Can you work these out from the model? Positions are in its coordinate system, mm. Face numbers are marked on the shaded views. A direction names the side the tool comes from. Coordinates: 2 decimals unless noted, no trailing zeros. Loops run counter-clockwise (first coordinate to the right, second up) from the corner with the lowest first, then second, coordinate; pieces in that order, holes last. Notation, with made-up numbers: (5, 31) -> (64, 31) arc R10 ccw to (64, 35) -> close; hole circle Ø7 at (-34.5, 77). An arc over 180 degrees is marked (long way). Use one line per item in the form item = value. Start each with the question number.
(1) On a 3-axis mill with a long thin cutter (end or side, diameter ignored), from which of +Z, -Z, +X, -X, +Y, -Y can I reach the whole of each face in a straight line? I mean the marked faces 4, 5, 6 and 7. Say none if no direction works.
(2) Imagine slicing it at A-A (y = -16). List the corners of the cut face in (x, z) for me, plus the area to 3 significant figures.
(3) I'm going to push flat-ended pins straight in: pin 1 (3 mm diameter, centred on y = -11, z = 16.01, fed in from -X); pin 2 (4 mm diameter, centred on y = -12.5, z = 12, fed in from +X); pin 3 (2 mm diameter, centred on x = 23, y = -13.5, fed in from +Z). Where does each tip first touch, or does it pass through?
(4) Thinking about a two-plate mould opening in X: for the marked faces 1, 2 and 3, which applies, released by +X, released by -X, zero draft, split by the parting line, or undercut?
(5) Imagine slicing it at C-C (x = 28). List the corners of the cut face in (y, z) for me.
(6) Imagine slicing it at B-B (z = 8). List the corners of the cut face in (x, y) for me, plus the area to 3 significant figures.
(7) Imagine slicing it at D-D (y = -11). List the corners of the cut face in (x, z) for me, plus the area to 3 significant figures.
(8) I need wall thicknesses on line 1 (X direction, y = -9.5, z = 23.5); line 2 (Z direction, x = 29.5, y = -10.75); line 3 (X direction, y = -2.5, z = 4.5). Which ranges of each line are inside material? Lowest first, please. Write a range as [from, to].
```python
from build123d import *

# Parameters (mm, degrees)
F0_W      = 50
F0_H      = 32
F1_DEPTH  = 24
F2_SIZE   = 4.5
F3_W      = 64.6181842312
F3_H      = 72.6516954601
F4_DEPTH  = 6.5
F6_DEPTH  = 13
F7_R      = 1.4
F8_DEPTH  = 5
F9_R      = 1.4
F10_DEPTH = 5
F11_R     = 1.4
F12_DEPTH = 5
F13_R     = 1.4
F14_DEPTH = 5
F15_R     = 1
F16_DEPTH = 5
F17_R     = 1
F18_DEPTH = 5
F19_R     = 1
F20_DEPTH = 5
F21_R     = 1
F22_DEPTH = 5
F23_R     = 1.1
F24_DEPTH = 25.4
F25_R     = 1.25
F26_DEPTH = 25.4
F27_R     = 1.25
F28_DEPTH = 25.4
F30_DEPTH = 25.4
F32_DEPTH = 25.4


# Not quite as in the source:
# - a feature names something its author has since deleted; it is built from what else it names


with BuildPart() as f1:
    # F0 (on Front) → F1 (new body)
    with BuildSketch(Plane.XZ):
        with Locations((25, 16)):
            Rectangle(F0_W, F0_H)
    extrude(amount=F1_DEPTH)

    # F2
    f2_edges = [f1.edges().sort_by_distance(p)[0] for p in [
        (50, -12, 0),
        (50, -12, 32),
        (50, 0, 16),
        (50, -24, 16),
        (0, -12, 32),
        (25, 0, 32),
        (25, -24, 32),
        (0, -12, 0),
        (0, 0, 16),
        (0, -24, 16),
        (25, 0, 0),
        (25, -24, 0),
    ]]
    chamfer(f2_edges, length=F2_SIZE)

    # F3 (on face) → F4 (cut)
    with BuildSketch(Plane.XZ.offset(24)):
        with Locations((22.701323498, 16.0673912615)):
            Rectangle(F3_W, F3_H)
    extrude(amount=-F4_DEPTH, mode=Mode.SUBTRACT)

    # F5 (on face) → F6 (cut)
    with BuildSketch(Plane.XZ.offset(17.5)):
        Polygon((4.5, 30), (2, 27.5), (2, 4.5), (4.5, 2), (45.5, 2), (48, 4.5), (48, 27.5), (45.5, 30), align=None)
    extrude(amount=-F6_DEPTH, mode=Mode.SUBTRACT)

    # F7 (on face) → F8 (join)
    with BuildSketch(Plane(origin=(38.75, 0, 38.75), x_dir=(0, 1, 0), z_dir=(0.7071067812, 0, 0.7071067812))):
        with Locations((-13.25, -12.7279220614)):
            Circle(F7_R)
        with Locations((-8.75, -12.7279220614)):
            Circle(F7_R)
    extrude(amount=F8_DEPTH)

    # F9 (on face) → F10 (join)
    with BuildSketch(Plane(origin=(22.75, 0, -22.75), x_dir=(0, 1, 0), z_dir=(0.7071067812, 0, -0.7071067812))):
        with Locations((-13.25, 35.3553390593)):
            Circle(F9_R)
        with Locations((-8.75, 35.3553390593)):
            Circle(F9_R)
    extrude(amount=F10_DEPTH)

    # F11 (on face) → F12 (join)
    with BuildSketch(Plane(origin=(2.25, 0, 2.25), x_dir=(0, -1, 0), z_dir=(-0.7071067812, 0, -0.7071067812))):
        with Locations((13.25, 0)):
            Circle(F11_R)
        with Locations((8.75, 0)):
            Circle(F11_R)
    extrude(amount=F12_DEPTH)

    # F13 (on face) → F14 (join)
    with BuildSketch(Plane(origin=(-13.75, 0, 13.75), x_dir=(0, -1, 0), z_dir=(-0.7071067812, 0, 0.7071067812))):
        with Locations((8.75, 22.6343975133)):
            Circle(F13_R)
        with Locations((13.25, 22.6343975133)):
            Circle(F13_R)
    extrude(amount=F14_DEPTH)

    # F15 (on face) → F16 (cut)
    with BuildSketch(Plane(origin=(42.2855339059, 0, 42.2855339059), x_dir=(0, 1, 0), z_dir=(0.7071067812, 0, 0.7071067812))):
        with Locations((-13.25, -12.7279220614)):
            Circle(F15_R)
        with Locations((-8.75, -12.7279220614)):
            Circle(F15_R)
    extrude(amount=-F16_DEPTH, mode=Mode.SUBTRACT)

    # F17 (on face) → F18 (cut)
    with BuildSketch(Plane(origin=(26.2855339059, 0, -26.2855339059), x_dir=(0, 1, 0), z_dir=(0.7071067812, 0, -0.7071067812))):
        with Locations((-13.25, 35.3553390593)):
            Circle(F17_R)
        with Locations((-8.75, 35.3553390593)):
            Circle(F17_R)
    extrude(amount=-F18_DEPTH, mode=Mode.SUBTRACT)

    # F19 (on face) → F20 (cut)
    with BuildSketch(Plane(origin=(-1.2855339059, 0, -1.2855339059), x_dir=(0, -1, 0), z_dir=(-0.7071067812, 0, -0.7071067812))):
        with Locations((13.25, 0)):
            Circle(F19_R)
        with Locations((8.75, 0)):
            Circle(F19_R)
    extrude(amount=-F20_DEPTH, mode=Mode.SUBTRACT)

    # F21 (on face) → F22 (cut)
    with BuildSketch(Plane(origin=(-17.2855339059, 0, 17.2855339059), x_dir=(0, -1, 0), z_dir=(-0.7071067812, 0, 0.7071067812))):
        with Locations((8.75, 22.6343975133)):
            Circle(F21_R)
        with Locations((13.25, 22.6343975133)):
            Circle(F21_R)
    extrude(amount=-F22_DEPTH, mode=Mode.SUBTRACT)

    # F23 (on face) → F24 (cut)
    with BuildSketch(Plane(origin=(0, 0, 0), x_dir=(0, -1, 0), z_dir=(-1, 0, 0))):
        with Locations((11, 16.0062)):
            Circle(F23_R)
    extrude(amount=-F24_DEPTH, mode=Mode.SUBTRACT)

    # F25 (on face) → F26 (cut)
    with BuildSketch(Plane(origin=(24.3333333333, 24.3333333333, 24.3333333333), x_dir=(-0.4082482905, 0.8164965809, -0.4082482905), z_dir=(0.5773502692, 0.5773502692, 0.5773502692))):
        with Locations((-33.0634771251, -12.7279220614)):
            Circle(F25_R)
    extrude(amount=-F26_DEPTH, mode=Mode.SUBTRACT)

    # F27 (on face) → F28 (cut)
    with BuildSketch(Plane(origin=(13.6666666667, 13.6666666667, -13.6666666667), x_dir=(-0.4082482905, 0.8164965809, 0.4082482905), z_dir=(0.5773502692, 0.5773502692, -0.5773502692))):
        with Locations((-19.7495318303, 35.3553390593)):
            Circle(F27_R)
    extrude(amount=-F28_DEPTH, mode=Mode.SUBTRACT)

    # F29 (on face) → F30 (cut)
    with BuildSketch(Plane(origin=(-7.6666666667, 7.6666666667, 7.6666666667), x_dir=(-0.8164965809, -0.4082482905, -0.4082482905), z_dir=(-0.5773502692, 0.5773502692, 0.5773502692))):
        with BuildLine():
            ThreePointArc((-12.8330958098, 23.027260035), (-14.5406275645, 22.5697282803), (-14.0830958098, 20.8621965255))
            Line((-14.0830958098, 20.8621965255), (-12.8330958098, 23.027260035))
        make_face()
        with BuildLine():
            Line((-12.8330958098, 23.027260035), (-14.0830958098, 20.8621965255))
            ThreePointArc((-14.0830958098, 20.8621965255), (-12.8330958098, 20.8621965255), (-12.2080958098, 21.9447282803))
            ThreePointArc((-12.2080958098, 21.9447282803), (-12.3755640551, 22.5697282803), (-12.8330958098, 23.027260035))
        make_face()
    extrude(amount=-F30_DEPTH, mode=Mode.SUBTRACT)

    # F31 (on face) → F32 (cut)
    with BuildSketch(Plane(origin=(3, -3, 3), x_dir=(-0.8164965809, -0.4082482905, 0.4082482905), z_dir=(-0.5773502692, 0.5773502692, -0.5773502692))):
        with BuildLine():
            ThreePointArc((1.0435586535, 0.3575669008), (0.4185586535, 1.4400986556), (-0.8314413465, 1.4400986556))
            Line((-0.8314413465, 1.4400986556), (0.4185586535, -0.7249648539))
            ThreePointArc((0.4185586535, -0.7249648539), (0.8760904083, -0.2674330992), (1.0435586535, 0.3575669008))
        make_face()
        with BuildLine():
            Line((0.4185586535, -0.7249648539), (-0.8314413465, 1.4400986556))
            ThreePointArc((-0.8314413465, 1.4400986556), (-1.2889731012, -0.2674330992), (0.4185586535, -0.7249648539))
        make_face()
    extrude(amount=-F32_DEPTH, mode=Mode.SUBTRACT)


solid = f1.part
```
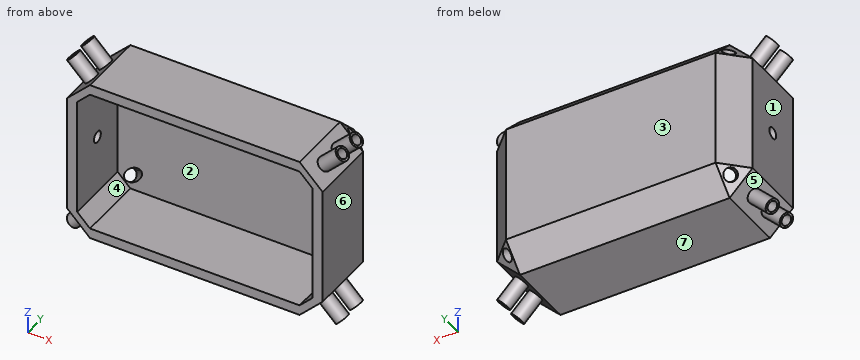
Worked out:
q1.face_4 = -Y
q1.face_5 = none
q1.face_6 = +X, +Y, -Y
q1.face_7 = -Z, +Y, -Y
q2.outline = (0, 4.5) -> (4.5, 0) -> (45.5, 0) -> (50, 4.5) -> (50, 27.5) -> (45.5, 32) -> (4.5, 32) -> (0, 27.5) -> close; hole (2, 4.5) -> (4.5, 2) -> (45.5, 2) -> (48, 4.5) -> (48, 27.5) -> (45.5, 30) -> (4.5, 30) -> (2, 27.5) -> close
q2.area = 284 mm2
q3.pin_1 = 0
q3.pin_2 = 50
q3.pin_3 = 32
q4.face_1 = released by -X
q4.face_2 = undercut
q4.face_3 = zero draft
q5.outline = (-17.5, 0) -> (-4.5, 0) -> (0, 4.5) -> (0, 27.5) -> (-4.5, 32) -> (-17.5, 32) -> (-17.5, 30) -> (-4.5, 30) -> (-4.5, 2) -> (-17.5, 2) -> close
q6.outline = (0, -17.5) -> (2, -17.5) -> (2, -4.5) -> (48, -4.5) -> (48, -17.5) -> (50, -17.5) -> (50, -4.5) -> (45.5, 0) -> (4.5, 0) -> (0, -4.5) -> close
q6.area = 257 mm2
q7.outline = (0, 4.5) -> (4.5, 0) -> (45.5, 0) -> (50, 4.5) -> (50, 27.5) -> (45.5, 32) -> (4.5, 32) -> (0, 27.5) -> (0, 17.11) -> (2, 17.11) -> (2, 27.5) -> (4.5, 30) -> (45.5, 30) -> (48, 27.5) -> (48, 4.5) -> (45.5, 2) -> (4.5, 2) -> (2, 4.5) -> (2, 14.91) -> (0, 14.91) -> close
q7.area = 280 mm2
q8.line_1 = [0, 2], [48, 50]
q8.line_2 = [0, 2], [30, 32]
q8.line_3 = [2, 2.93], [4.57, 44.96], [47.23, 48]
